from build123d import *

# Parameters (mm, degrees)
F0_W     = 200
F0_H     = 100
F1_DEPTH = 21.6
F2_R     = 4
F4_DEPTH = 1
F5_R     = 8.5
F6_DEPTH = 10
F7_R     = 5
F8_W     = 24
F8_H     = 30.4
F9_DEPTH = 10


with BuildPart() as f1:
    # F0 (on Right) → F1 (new body, symmetric)
    with BuildSketch(Plane.YZ):
        with Locations((20.360822, 10.377156)):
            Rectangle(F0_W, F0_H)
    extrude(amount=F1_DEPTH, both=True)

    # F2
    f2_edges = [f1.edges().sort_by_distance(p)[0] for p in [
        (0, -79.639178, 60.377156),
        (-21.6, -79.639178, 10.377156),
        (-21.6, 20.360822, 60.377156),
        (21.6, 20.360822, 60.377156),
        (21.6, -79.639178, 10.377156),
        (0, -79.639178, -39.622844),
        (-21.6, 20.360822, -39.622844),
        (21.6, 20.360822, -39.622844),
        (21.6, 120.360822, 10.377156),
        (0, 120.360822, -39.622844),
        (-21.6, 120.360822, 10.377156),
        (0, 120.360822, 60.377156),
    ]]
    fillet(f2_edges, radius=F2_R)

    # F3 (on face) → F4 (cut)
    with BuildSketch(Plane.YZ.offset(21.6)):
        with BuildLine():
            Line((106.260822, -26.622844), (106.360822, -26.622844))
            ThreePointArc((106.360822, -26.622844), (107.775035, -26.037058), (108.360822, -24.622844))
            Line((108.360822, -24.622844), (108.360822, -20.622844))
            ThreePointArc((108.360822, -20.622844), (107.775035, -19.208631), (106.360822, -18.622844))
            Line((106.360822, -18.622844), (106.260822, -18.622844))
            ThreePointArc((106.260822, -18.622844), (104.846608, -19.208631), (104.260822, -20.622844))
            Line((104.260822, -20.622844), (104.260822, -24.622844))
            ThreePointArc((104.260822, -24.622844), (104.846608, -26.037058), (106.260822, -26.622844))
        make_face()
    extrude(amount=-F4_DEPTH, mode=Mode.SUBTRACT)

    # F5 (on face) → F6 (join)
    with BuildSketch(Plane(origin=(0, 120.360822, 0), x_dir=(-1, 0, 0), z_dir=(0, 1, 0))):
        with Locations((0, -6.122844)):
            Circle(F5_R)
    extrude(amount=F6_DEPTH)

    # F7
    f7_edges = [f1.edges().sort_by_distance(p)[0] for p in [
        (8.5, 130.360822, -6.122844),
    ]]
    fillet(f7_edges, radius=F7_R)

    # F8 (on face) → F9 (cut)
    with BuildSketch(Plane.XZ.offset(79.639178)):
        with Locations((0, -7.622844)):
            Rectangle(F8_W, F8_H)
        Polygon((-9, -19.822844), (-9, 4.177156), (3.575129, 4.386477), (9, -1.319719), (9, -14.319719), (3.576871, -19.822844), align=None, mode=Mode.SUBTRACT)
    extrude(amount=-F9_DEPTH, mode=Mode.SUBTRACT)


solid = f1.part
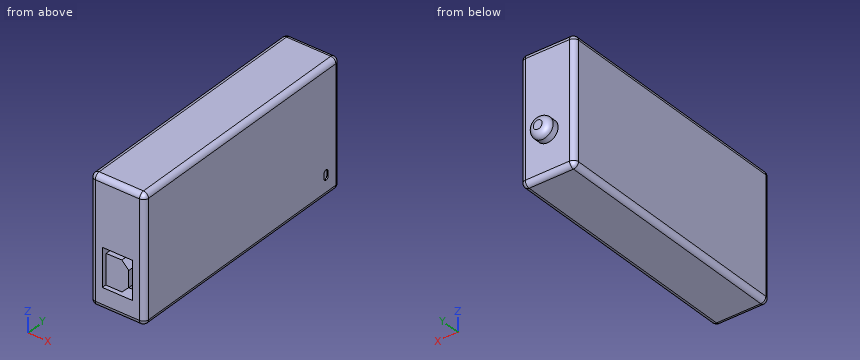
Can you work these out from the model? Positions are in its coordinate system, mm. Give positions to 0.01 mm unless a question says otherwise; leave off trailing zeros. Loops run counter-clockwise (first coordinate to the right, second up) from the corner with the lowest first, then second, coordinate; pieces in that order, holes last. Notation, with made-up numbers: M 55.5,19 L 62.5,19 A4 ccw 62.5,26 Z; hole C -37.5,-35.75 d4. An arc over 180 degrees is marked long. One line per item, written item: value.
1) Imagine slicing it at A-A on z = 35. Write out the boundary of the cut face in (x, y).
Geometry check:
outline: M -21.6,-75.64 A4 ccw -17.6,-79.64 L 17.6,-79.64 A4 ccw 21.6,-75.64 L 21.6,116.36 A4 ccw 17.6,120.36 L -17.6,120.36 A4 ccw -21.6,116.36 Z
2) I'm going to push flat-ended pins straight in: pin 1 (11 mm diameter, centred on y = -76.5, z = -3, fed in from -X); pin 2 (0.5 mm diameter, centred on x = 21.5, z = -22, fed in from +Y); pin 3 (12 mm diameter, centred on x = 12.5, z = -24, fed in from +Y); pin 4 (0.8 mm diameter, centred on x = 21, z = -22.5, fed in from -Y). Where does each tip first touch, or does it pass through?
Geometry check:
pin 1: stops at x = -21.6
pin 2: stops at y = 118
pin 3: stops at y = 120.36
pin 4: stops at y = -78.28
3) Please list where these lines run through material, in increasing order: line 1 (Y direction, x = 18, z = 51); line 2 (Y direction, x = 3, z = -17.5); line 3 (X direction, y = 122, z = 0).
Geometry check:
line 1: y = -79.62 to 120.34
line 2: y = -79.64 to 120.36
line 3: x = -5.9 to 5.9
